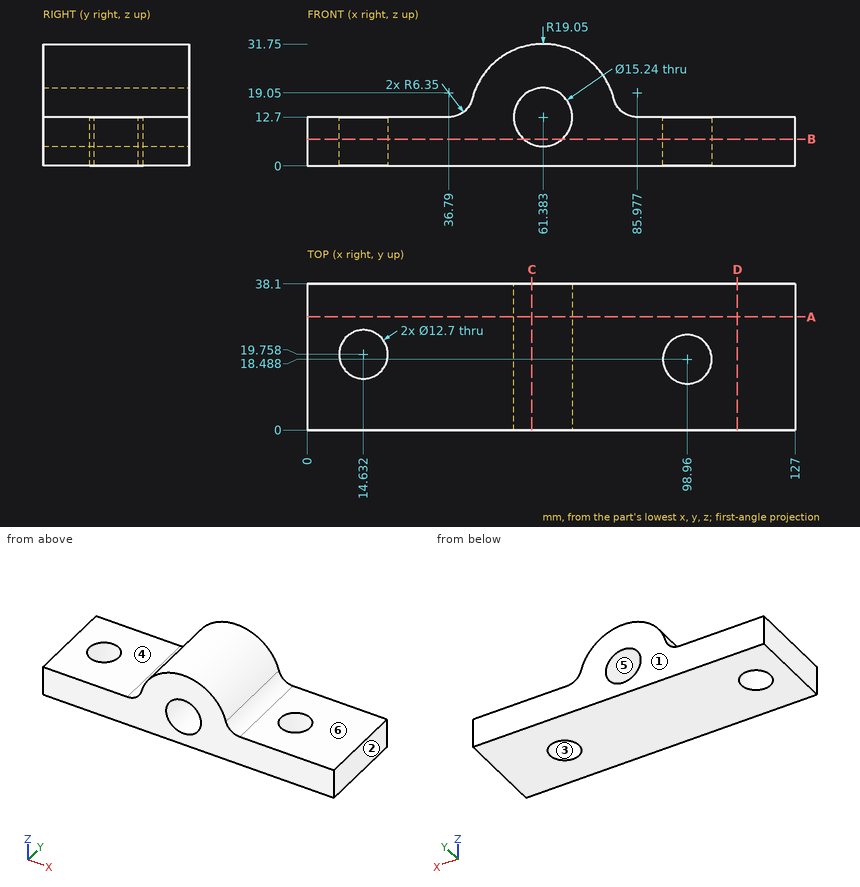
Input: dimensioned drawing with shaded views. Units: mm. Origin: part minimum x, y, z. A direction names the side the tool comes from. Coordinates: 2 decimals unless noted, no trailing zeros. Order: outer loops, then holes, each group sorted by start corner. A loop starts at its lowest first (then second) coordinate and runs counter-clockwise, first axis right, second up.
Item 1: Access query for the marked faces 4, 5 and 6. Directions: +Z, -Z, +X, -X, +Y, -Y. A direction counts if a zero-diameter tool reaches every point of the face in a straight line with its end or side. Return the directions, or none.
Answer:
face 4: +Z, -X, +Y, -Y
face 5: +Y, -Y
face 6: +Z, +X, +Y, -Y
Item 2: Draft query along X for the marked faces 1, 2 and 3. Return one class per face: released by +X, released by -X, zero draft, split by the parting line, or undercut.
Answer:
face 1: zero draft
face 2: released by +X
face 3: undercut
Item 3: Section query D-D (x = 112). Output: boundary loops of the cut face in (y, z).
Answer:
outline: (0, 0) - (38.1, 0) - (38.1, 12.7) - (0, 12.7) - close
Item 4: Material intervals for line 1 along Z through (x, y) = (35, 35); line 2 along X through (y, z) = (10, 14) (1 decimal); line 3 along X through (y, z) = (34, 7) (1 decimal), sorted ascending.
Answer:
line 1: z = 0 to 12.7
line 2: x = 40.6 to 53.9, 68.9 to 82.1
line 3: x = 0 to 56.3, 66.4 to 127
Item 5: Section query B-B (z = 7). Output: boundary loops of the cut face in (x, y), then the cut area to 3 significant figures.
Answer:
outline: (0, 0) - (56.33, 0) - (56.33, 38.1) - (0, 38.1) - close; (66.44, 0) - (127, 0) - (127, 38.1) - (66.44, 38.1) - close; hole circle Ø12.7 at (14.63, 19.76); hole circle Ø12.7 at (98.96, 18.49)
area: 4,200 mm2
Item 6: Section query C-C (x = 58.5). Output: boundary loops of the cut face in (y, z).
Answer:
outline: (0, 0) - (38.1, 0) - (38.1, 5.65) - (0, 5.65) - close; (0, 19.75) - (38.1, 19.75) - (38.1, 31.53) - (0, 31.53) - close
Item 7: Section query A-A (y = 29.5). Output: boundary loops of the cut face in (x, z).
Answer:
outline: (0, 0) - (127, 0) - (127, 12.7) - (85.98, 12.7) arc R6.35 cw to (79.83, 17.46) arc R19.05 ccw to (42.94, 17.46) arc R6.35 cw to (36.79, 12.7) - (0, 12.7) - close; hole circle Ø15.24 at (61.38, 12.7)
Item 8: Contact query for flat-ended pins moving along their axis: P1, Ø10, axis at x = 93, z = 21, coming from the -Y side; P2, Ø5, axis at y = 8.5, z = 20, coming from the -X side; P3, Ø18.5, axis at x = 14.5, y = 27.5, coming from the +Z side. Output: stop coordinate, or through.
Answer:
P1: passes through
P2: stops at x = 42.95
P3: stops at z = 12.7
